Check sheet for the modelled part. Datum: model origin and axes. Units: mm. A direction names the side the tool comes from. Round coordinates to 2 decimals unless told otherwise and drop trailing zeros. Loops run counter-clockwise (first coordinate to the right, second up) from the corner with the lowest first, then second, coordinate; pieces in that order, holes last. Notation, with made-up numbers: (47, -22) -> (74, -22) arc R29 cw to (74, 14) -> close; hole circle Ø4 at (72.25, 30.5). An arc over 180 degrees is marked (long way). One line per question, with ' | ' between items.
```python
from build123d import *

# Parameters (mm, degrees)
F0_R      = 22.225
F1_DEPTH  = 44.45
F2_R      = 5.08
F3_T      = -2.54
F4_W      = 10.4627240348
F4_H      = 5.334
F5_DEPTH  = 2.794
F6_SIZE   = 1.27
F7_W      = 12.1457316697
F7_H      = 17.4408461899
F8_DEPTH  = 5.08
F9_R      = 0.381
F10_DEPTH = 6.35
F11_R     = 0.381
F12_DEPTH = 6.35
F13_R     = 1.016


with BuildPart() as f1:
    # F0 (on Top) → F1 (new body)
    with BuildSketch(Plane.XY):
        Circle(F0_R)
    extrude(amount=F1_DEPTH)

    # F2
    f2_edges = [f1.edges().sort_by_distance(p)[0] for p in [
        (-22.225, 0, 0),
    ]]
    fillet(f2_edges, radius=F2_R)

    # F3
    f3_openings = [f1.faces().sort_by_distance(p)[0] for p in [
        (0, 0, 44.45),
    ]]
    offset(amount=F3_T, openings=f3_openings)

    # F4 (on face) → F5 (cut)
    with BuildSketch(Plane.XY.offset(44.45)):
        with Locations((19.685, 0)):
            Rectangle(F4_W, F4_H)
    extrude(amount=-F5_DEPTH, mode=Mode.SUBTRACT)

    # F6
    f6_edges = [f1.edges().sort_by_distance(p)[0] for p in [
        (-19.685, 0, 44.45),
    ]]
    chamfer(f6_edges, length=F6_SIZE)

    # F7 (on face) → F8 (cut)
    with BuildSketch(Plane.XY.offset(44.45)):
        with Locations((-22.225, 0)):
            Rectangle(F7_W, F7_H)
    extrude(amount=-F8_DEPTH, mode=Mode.SUBTRACT)

    # F9 (on face) → F10 (cut)
    with BuildSketch(Plane(origin=(0, -8.7204230949, 0), x_dir=(-1, 0, 0), z_dir=(0, 1, 0))):
        with Locations((19.0542973118, 41.91)):
            Circle(F9_R)
    extrude(amount=-F10_DEPTH, mode=Mode.SUBTRACT)

    # F11 (on face) → F12 (cut)
    with BuildSketch(Plane.XZ.offset(-8.7204230949)):
        with Locations((-19.0542973118, 41.91)):
            Circle(F11_R)
    extrude(amount=-F12_DEPTH, mode=Mode.SUBTRACT)

    # F13
    f13_edges = [f1.edges().sort_by_distance(p)[0] for p in [
        (-19.748509, 8.720423, 44.45),
        (-19.748509, -8.720423, 44.45),
        (-18.352286, -8.720423, 43.813764),
        (-18.352286, 8.720423, 43.813764),
    ]]
    fillet(f13_edges, radius=F13_R)


solid = f1.part
```
(1) Set-up check for faces 4 (the face through (-20, 0, 39.37)), 5 (the face through (21, -2.667, 43)), 6 (the face through (5.6, -20.4, 44.45)), 7 (the face through (3.709, 19.539, 43.383)): record each of +Z, -Z, +X, -X, +Y, -Y from which the full face is reachable in a straight line by a thin tool's end or side.
Answer:
face 4: +Z, -X | face 5: +Z, +X, -X | face 6: +Z, +X, -X, +Y, -Y | face 7: +Z
(2) Sectioned sample at A-A, the plane y = 0. Record the cut outline in (x, z) (3 decimals).
Answer:
outline: (-22.225, 5.08) arc R5.08 ccw to (-17.145, 0) -> (17.145, 0) arc R5.08 ccw to (22.225, 5.08) -> (22.225, 41.656) -> (19.685, 41.656) -> (19.685, 5.08) arc R2.54 cw to (17.145, 2.54) -> (-17.145, 2.54) arc R2.54 cw to (-19.685, 5.08) -> (-19.685, 39.37) -> (-22.225, 39.37) -> close
(3) Sectioned sample at B-B, the plane x = 0. Record the cut outline in (y, z) (3 decimals), and give its area (3 significant figures).
Answer:
outline: (-22.225, 5.08) arc R5.08 ccw to (-17.145, 0) -> (17.145, 0) arc R5.08 ccw to (22.225, 5.08) -> (22.225, 44.45) -> (20.955, 44.45) -> (19.685, 43.18) -> (19.685, 5.08) arc R2.54 cw to (17.145, 2.54) -> (-17.145, 2.54) arc R2.54 cw to (-19.685, 5.08) -> (-19.685, 43.18) -> (-20.955, 44.45) -> (-22.225, 44.45) -> close | area: 316 mm2
(4) Scan lines: probe 1 along X at (y, z) = (0, 26) (3 decimals); probe 2 along X at (y, z) = (9.4, 41.91). Record each from-to range of solid material in increasing order.
Answer:
probe 1: x = -22.225 to -19.685, 19.685 to 22.225 | probe 2: x = -20.14 to -19.44, -18.67 to -17.3, 17.3 to 20.14
(5) Go/stop test with flat-tipped pins: pin 1 (6 mm diameter, centred on x = 13.5, z = 32.5, fed in from +Y); pin 2 (3 mm diameter, centred on x = -19, z = 41.5, fed in from -Y); pin 3 (0.8 mm diameter, centred on x = 21, z = 42.5, fed in from -Y). Record where each tip stops, or that it passes through.
Answer:
pin 1: stops at y = 19.59 | pin 2: stops at y = -13.7 | pin 3: stops at y = -8.34
(6) Sectioned sample at C-C, the plane z = 40. Record the cut outline in (x, y) (3 decimals), and give its area (3 significant figures).
Answer:
outline: (-20.443, -8.72) arc R22.225 ccw (long way) to (-20.443, 8.72) -> (-17.648, 8.72) arc R19.685 cw (long way) to (-17.648, -8.72) -> close | area: 289 mm2
(7) Mould release check, pull along X, two halves, no side actions. Record for faces 1 (the face through (0, 0, 0)), 2 (the face through (21.199, 6.676, 24.489)), 3 (the face through (0, 0, 2.54)): +X half, -X half, draft (parallel to the pull), parting line (faces both ways), or undercut.
Answer:
face 1: draft | face 2: parting line | face 3: undercut
